Model file for the job. Use its own axes, mm. Face numbers are marked on the shaded views. A direction names the side the tool comes from. Round coordinates to 2 decimals unless told otherwise and drop trailing zeros. Write each loop counter-clockwise with the first axis right and the second up, starting at its lowest first coordinate (ties: lowest second). Pieces come first, ordered by that corner, then holes.
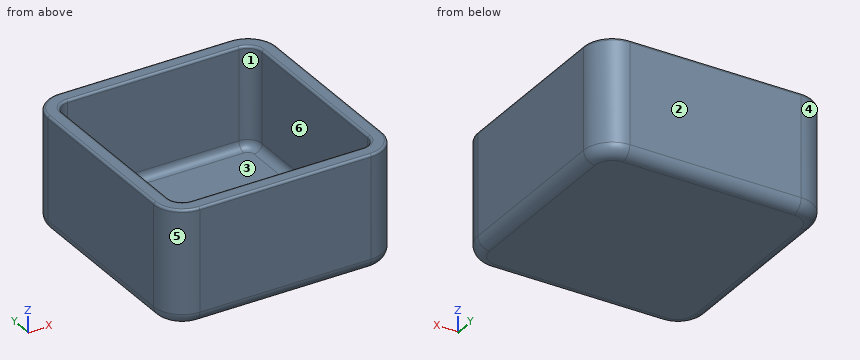
```python
from build123d import *

# Parameters (mm, degrees)
F1_DEPTH = 25.4
F3_DEPTH = 22.225
F4_R     = 2.54
F5_R     = 1.778
F6_R     = 0.508


with BuildPart() as f1:
    # F0 (on Top) → F1 (new body)
    with BuildSketch(Plane.XY):
        with BuildLine():
            ThreePointArc((25.4, 22.2595424831), (23.5401280605, 26.7496705436), (19.05, 28.6095424831))
            Line((19.05, 28.6095424831), (-19.05, 28.6095424831))
            ThreePointArc((-19.05, 28.6095424831), (-23.5401280605, 26.7496705436), (-25.4, 22.2595424831))
            Line((-25.4, 22.2595424831), (-25.4, -15.8404575169))
            ThreePointArc((-25.4, -15.8404575169), (-23.5401280605, -20.3305855774), (-19.05, -22.1904575169))
            Line((-19.05, -22.1904575169), (19.05, -22.1904575169))
            ThreePointArc((19.05, -22.1904575169), (23.5401280605, -20.3305855774), (25.4, -15.8404575169))
            Line((25.4, -15.8404575169), (25.4, 22.2595424831))
        make_face()
    extrude(amount=F1_DEPTH)

    # F2 (on face) → F3 (cut)
    with BuildSketch(Plane.XY.offset(25.4)):
        with BuildLine():
            Line((19.05, 25.4345424831), (-19.05, 25.4345424831))
            ThreePointArc((-19.05, 25.4345424831), (-21.2950640303, 24.5046065134), (-22.225, 22.2595424831))
            Line((-22.225, 22.2595424831), (-22.225, -15.8404575169))
            ThreePointArc((-22.225, -15.8404575169), (-21.2950640303, -18.0855215472), (-19.05, -19.0154575169))
            Line((-19.05, -19.0154575169), (19.05, -19.0154575169))
            ThreePointArc((19.05, -19.0154575169), (21.2950640303, -18.0855215472), (22.225, -15.8404575169))
            Line((22.225, -15.8404575169), (22.225, 22.2595424831))
            ThreePointArc((22.225, 22.2595424831), (21.2950640303, 24.5046065134), (19.05, 25.4345424831))
        make_face()
    extrude(amount=-F3_DEPTH, mode=Mode.SUBTRACT)

    # F4
    f4_edges = [f1.edges().sort_by_distance(p)[0] for p in [
        (23.540128, -20.330586, 0),
        (25.4, 3.209542, 0),
        (23.540128, 26.749671, 0),
        (0, 28.609542, 0),
        (-23.540128, 26.749671, 0),
        (-25.4, 3.209542, 0),
        (-23.540128, -20.330586, 0),
        (0, -22.190458, 0),
    ]]
    fillet(f4_edges, radius=F4_R)

    # F5
    f5_edges = [f1.edges().sort_by_distance(p)[0] for p in [
        (0, 25.434542, 3.175),
        (-21.295064, 24.504607, 3.175),
        (-22.225, 3.209542, 3.175),
        (-21.295064, -18.085522, 3.175),
        (0, -19.015458, 3.175),
        (21.295064, -18.085522, 3.175),
        (22.225, 3.209542, 3.175),
        (21.295064, 24.504607, 3.175),
    ]]
    fillet(f5_edges, radius=F5_R)

    # F6
    f6_edges = [f1.edges().sort_by_distance(p)[0] for p in [
        (23.540128, -20.330586, 25.4),
        (0, -22.190458, 25.4),
        (25.4, 3.209542, 25.4),
        (-23.540128, -20.330586, 25.4),
        (23.540128, 26.749671, 25.4),
        (-25.4, 3.209542, 25.4),
        (0, 28.609542, 25.4),
        (-23.540128, 26.749671, 25.4),
        (0, 25.434542, 25.4),
        (-21.295064, 24.504607, 25.4),
        (-22.225, 3.209542, 25.4),
        (-21.295064, -18.085522, 25.4),
        (0, -19.015458, 25.4),
        (21.295064, -18.085522, 25.4),
        (22.225, 3.209542, 25.4),
        (21.295064, 24.504607, 25.4),
    ]]
    fillet(f6_edges, radius=F6_R)


solid = f1.part
```
1) Cut at B-B on x = 0.5. List the corners of the cut face in (y, z) (3 decimals), and give its area (3 significant figures).
2) Wall check: probe 1 along Y at (x, z) = (-6.5, 13.25); probe 2 along X at (y, z) = (-10.5, 9.5) (3 decimals); probe 3 along Z at (x, y) = (17, -8) (3 decimals). Give the ranges that are in metal, low to high.
3) Pull direction X, two halves, no side cores. Call the marked faces 1, 2, 3 and 4: released by +X, released by -X, zero draft, split by the parting line, or undercut.
4) Cut at C-C on y = 21. List the corners of the cut face in (x, z) (3 decimals), and give its area (3 significant figures).
5) Cut at A-A on z = 17.75. List the corners of the cut face in (x, y) (3 decimals).
6) Which spindle directions (+Z, -Z, +X, -X, +Y, -Y) get a long thin tool onto all of the face, cutting with end or side? Do the marked faces 5 and 6. Say none if no direction does.
7) Flat gauge pin, fed straight in: pin 1 Ø8 at (x, y) = (-11, 12.5) entering from +Z (3 decimals). Where does the tip first touch, or does it go through?
Result sheet:
1. outline: (-22.19, 2.54) arc R2.54 ccw to (-19.65, 0) - (26.07, 0) arc R2.54 ccw to (28.61, 2.54) - (28.61, 24.892) arc R0.508 ccw to (28.102, 25.4) - (25.943, 25.4) arc R0.508 ccw to (25.435, 24.892) - (25.435, 4.953) arc R1.778 cw to (23.657, 3.175) - (-17.237, 3.175) arc R1.778 cw to (-19.015, 4.953) - (-19.015, 24.892) arc R0.508 ccw to (-19.523, 25.4) - (-21.682, 25.4) arc R0.508 ccw to (-22.19, 24.892) - close
1. area: 301 mm2
2. probe 1: y = -22.19 to -19.02, 25.43 to 28.61
2. probe 2: x = -25.4 to -22.225, 22.225 to 25.4
2. probe 3: z = 0 to 3.175
3. face 1: undercut
3. face 2: zero draft
3. face 3: undercut
3. face 4: released by -X
4. outline: (-25.4, 2.54) arc R2.54 ccw to (-22.86, 0) - (22.86, 0) arc R2.54 ccw to (25.4, 2.54) - (25.4, 24.892) arc R0.508 ccw to (24.892, 25.4) - (22.733, 25.4) arc R0.508 ccw to (22.225, 24.892) - (22.225, 4.953) arc R1.778 cw to (20.447, 3.175) - (-20.447, 3.175) arc R1.778 cw to (-22.225, 4.953) - (-22.225, 24.892) arc R0.508 ccw to (-22.733, 25.4) - (-24.892, 25.4) arc R0.508 ccw to (-25.4, 24.892) - close
4. area: 301 mm2
5. outline: (-25.4, -15.84) arc R6.35 ccw to (-19.05, -22.19) - (19.05, -22.19) arc R6.35 ccw to (25.4, -15.84) - (25.4, 22.26) arc R6.35 ccw to (19.05, 28.61) - (-19.05, 28.61) arc R6.35 ccw to (-25.4, 22.26) - close; hole (-22.225, -15.84) arc R3.175 ccw to (-19.05, -19.015) - (19.05, -19.015) arc R3.175 ccw to (22.225, -15.84) - (22.225, 22.26) arc R3.175 ccw to (19.05, 25.435) - (-19.05, 25.435) arc R3.175 ccw to (-22.225, 22.26) - close
6. face 5: +Z, -Z, -X, -Y
6. face 6: +Z
7. pin 1: stops at z = 3.175
